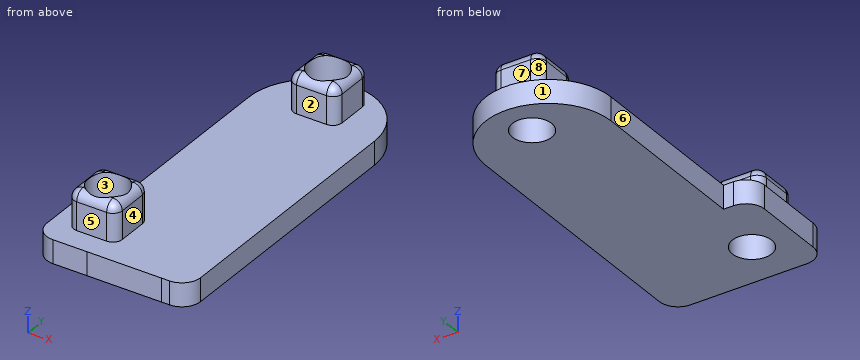
```python
from build123d import *

# Parameters (mm, degrees)
BOSS_EXTRUDE1_DEPTH = 2.5
SKETCH1_3_W         = 5.2
SKETCH1_3_H         = 5.2
BOSS_EXTRUDE2_DEPTH = 6.5
FILLET1_R           = 2
FILLET2_R           = 1
SKETCH2_R           = 2.1
CUT_EXTRUDE1_DEPTH  = 7.5


with BuildPart() as part:
    # Sketch1 → Boss-Extrude1 (new body)
    with BuildSketch(Plane(origin=(0, 0, 0), x_dir=(0, 1, 0), z_dir=(0, 0, 1))):
        with BuildLine():
            Line((-7.649421348, 9.749384529), (-7.649421348, 4.119353309))
            Line((-7.649421348, 4.119353309), (-7.652407104, -3.880646133))
            Line((-7.652407104, -3.880646133), (-7.652407104, -6.7))
            Line((-7.652407104, -6.7), (22, -6.7))
            ThreePointArc((22, -6.7), (28.7, 0), (22, 6.7))
            Line((22, 6.7), (4.1, 6.7))
            Line((4.1, 6.7), (4.1, 9.744999415))
            Line((4.1, 9.744999415), (-7.649421348, 9.749384529))
        make_face()
    extrude(amount=BOSS_EXTRUDE1_DEPTH)

    # Sketch1<3> → Boss-Extrude2 (add)
    with BuildSketch(Plane(origin=(0, 0, 0), x_dir=(0, 1, 0), z_dir=(0, 0, 1))):
        with Locations((24.6, 0)):
            Rectangle(SKETCH1_3_W, SKETCH1_3_H)
        with Locations((-2.6, 5.25)):
            Rectangle(SKETCH1_3_W, SKETCH1_3_H)
    extrude(amount=BOSS_EXTRUDE2_DEPTH)

    # Fillet1
    fillet1_edges = [part.edges().sort_by_distance(p)[0] for p in [
        (6.7, -7.652407104, 1.25),
        (-9.749384529, -7.649421348, 1.25),
        (-9.744999415, 4.1, 1.25),
    ]]
    fillet(fillet1_edges, radius=FILLET1_R)

    # Fillet2
    fillet2_edges = [part.edges().sort_by_distance(p)[0] for p in [
        (-2.65, -5.2, 4.5),
        (-2.65, -2.6, 6.5),
        (-2.65, 0, 4.5),
        (-7.85, 0, 4.5),
        (-7.85, -5.2, 4.5),
        (-5.25, -5.2, 6.5),
        (-5.25, 0, 6.5),
        (-7.85, -2.6, 6.5),
        (2.6, 22, 4.5),
        (2.6, 27.2, 4.5),
        (-2.6, 27.2, 4.5),
        (-2.6, 24.6, 6.5),
        (-2.6, 22, 4.5),
        (0, 22, 6.5),
        (2.6, 24.6, 6.5),
        (0, 27.2, 6.5),
    ]]
    fillet(fillet2_edges, radius=FILLET2_R)

    # Sketch2 → Cut-Extrude1 (cut)
    with BuildSketch(Plane.XY.offset(6.5)):
        with Locations((-5.25, -2.6)):
            Circle(SKETCH2_R)
        with Locations((0, 24.6)):
            Circle(SKETCH2_R)
    extrude(amount=-CUT_EXTRUDE1_DEPTH, mode=Mode.SUBTRACT)


solid = part.part
```
Input: part model. Units: mm. Frame: model coordinates. Face numbers are marked on the shaded views. A direction names the side the tool comes from. Give positions to 0.01 mm unless a question says otherwise; leave off trailing zeros. Loops run counter-clockwise (first coordinate to the right, second up) from the corner with the lowest first, then second, coordinate; pieces in that order, holes last.
1) Section query B-B on y = 24.6. Return the cut outline in (x, z).
A:
outline: (-6.17, 0) - (-2.1, 0) - (-2.1, 6.37) arc R1 ccw to (-2.6, 5.5) - (-2.6, 2.5) - (-6.17, 2.5) - close; (2.1, 0) - (6.17, 0) - (6.17, 2.5) - (2.6, 2.5) - (2.6, 5.5) arc R1 ccw to (2.1, 6.37) - close
2) Section query D-D on y = 3. Return the cut outline in (x, z).
A:
outline: (-9.53, 0) - (6.7, 0) - (6.7, 2.5) - (-9.53, 2.5) - close
3) Section query A-A on z = 4.25. Return the cut outline in (x, y), and give its area (3 significant figures).
A:
outline: (-7.85, -4.2) arc R1 ccw to (-6.85, -5.2) - (-3.65, -5.2) arc R1 ccw to (-2.65, -4.2) - (-2.65, -1) arc R1 ccw to (-3.65, 0) - (-6.85, 0) arc R1 ccw to (-7.85, -1) - close; (-2.6, 23) arc R1 ccw to (-1.6, 22) - (1.6, 22) arc R1 ccw to (2.6, 23) - (2.6, 26.2) arc R1 ccw to (1.6, 27.2) - (-1.6, 27.2) arc R1 ccw to (-2.6, 26.2) - close; hole circle Ø4.2 at (-5.25, -2.6); hole circle Ø4.2 at (0, 24.6)
area: 24.7 mm2
4) Section query C-C on x = -1. Return the cut outline in (y, z), and give its area (3 significant figures).
A:
outline: (-7.65, 0) - (22.75, 0) - (22.75, 6.47) arc R1 ccw to (22, 5.5) - (22, 2.5) - (-7.65, 2.5) - close; (26.45, 0) - (28.62, 0) - (28.62, 2.5) - (27.2, 2.5) - (27.2, 5.5) arc R1 ccw to (26.45, 6.47) - close
area: 87.1 mm2
5) Mould query, pull axis Y, two halves, no side actions, for the marked faces 1, 2 and 3. Classes: released by +Y, released by -Y, zero draft, split by the parting line, or undercut.
A:
face 1: released by +Y
face 2: released by -Y
face 3: undercut
6) Reachability of the marked faces 4, 5, 6, 7 and 8 from +Z, -Z, +X, -X, +Y, -Y: full face, straight path, thin tool, end or side. Return the list, or none.
A:
face 4: +Z, +X, +Y, -Y
face 5: +Z, +X, -X, -Y
face 6: +Z, -Z, -X, +Y
face 7: +Z, +X, -X, +Y
face 8: +Z, -X, +Y
7) Contact query for flat-ended pins moving along their axis: pin 1 (1.5 mm diameter, centred on x = -4.5, z = 3.5, fed in from +Y); pin 2 (0.8 mm diameter, centred on x = -5, z = 1.5, fed in from -Y); pin 3 (0.8 mm diameter, centred on x = -7.5, z = 0.5, fed in from +Y); pin 4 (2.5 mm diameter, centred on x = -5.25, y = -2.6, fed in from -Z). Output: stop coordinate, or through.
A:
pin 1: stops at y = 0
pin 2: stops at y = -7.65
pin 3: stops at y = 4.1
pin 4: passes through
8) Line query: L1, parallel to Y at x = 0, z = 2.75; L2, parallel to X at y = -2.6, z = 4.25; L3, parallel to Y at x = -5.25, z = 4.5. Output: solid intervals per line, ascending.
A:
L1: y = 22 to 22.5, 26.7 to 27.2
L2: x = -7.85 to -7.35, -3.15 to -2.65
L3: y = -5.2 to -4.7, -0.5 to 0
